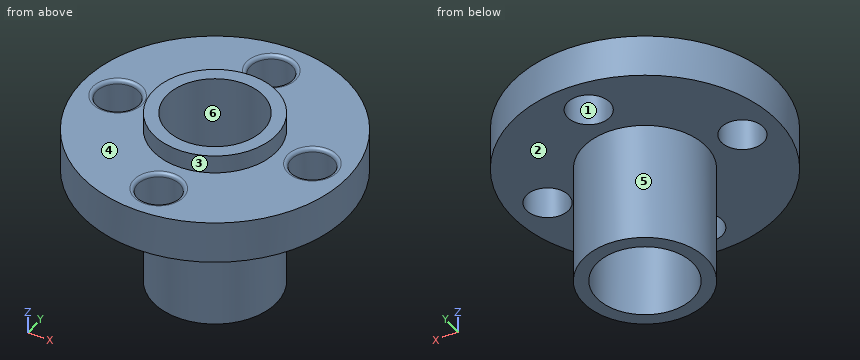
```python
from build123d import *

# Parameters (mm, degrees)
SKETCH1_R                = 11
SKETCH1_R_2              = 5.1
SKETCH1_R_3              = 1.75
BOSS_EXTRUDE1_DEPTH      = 3.5
BOSS_EXTRUDE2_DEPTH      = 1.5
BOSS_EXTRUDE2_DEPTH_BACK = 13.5
SKETCH2_R                = 5.1
SKETCH2_R_2              = 4
FILLET2_R                = 0.3


with BuildPart() as part:
    # Sketch1 → Boss-Extrude1 (new body)
    with BuildSketch(Plane.XY):
        Circle(SKETCH1_R)
        Circle(SKETCH1_R_2, mode=Mode.SUBTRACT)
        with Locations((0, 8)):
            Circle(SKETCH1_R_3, mode=Mode.SUBTRACT)
        with Locations((8, 0)):
            Circle(SKETCH1_R_3, mode=Mode.SUBTRACT)
        with Locations((0, -8)):
            Circle(SKETCH1_R_3, mode=Mode.SUBTRACT)
        with Locations((-8, 0)):
            Circle(SKETCH1_R_3, mode=Mode.SUBTRACT)
    extrude(amount=-BOSS_EXTRUDE1_DEPTH)

    # Sketch2 → Boss-Extrude2 (add, two sides: drawn at the far end of the back side and taken through both)
    with BuildSketch(Plane.XY.offset(-BOSS_EXTRUDE2_DEPTH_BACK)):
        Circle(SKETCH2_R)
        Circle(SKETCH2_R_2, mode=Mode.SUBTRACT)
    extrude(amount=BOSS_EXTRUDE2_DEPTH + BOSS_EXTRUDE2_DEPTH_BACK)

    # Fillet2
    fillet2_edges = [part.edges().sort_by_distance(p)[0] for p in [
        (6.25, 0, 0),
        (-1.75, -8, 0),
        (-9.75, 0, 0),
        (-1.75, 8, 0),
    ]]
    fillet(fillet2_edges, radius=FILLET2_R)


solid = part.part
```
The listing builds one solid part. Answer for the finished solid, in the listing's coordinates (mm). Face numbers are marked on the shaded views. A direction names the side the tool comes from. Round coordinates to 2 decimals unless told otherwise and drop trailing zeros. Order: outer loops, then holes, each group sorted by start corner. A loop starts at its lowest first (then second) coordinate and runs counter-clockwise, first axis right, second up. Notation, with made-up numbers: (-26.5, 43.5) - (12.5, 43.5) arc R33 ccw to (12.5, 74.5) - close; hole circle Ø11 at (33.25, 16). An arc over 180 degrees is marked (long way). Put each result on its own line as item: value. Start each with the question number.
(1) Straight lines are drawn through the part: probe 1 along Y at (x, z) = (0, -1.75); probe 2 along Z at (x, y) = (-4, 6.5); probe 3 along Y at (x, z) = (0, -8.5). For each, find the intervals that lie inside material, in ascending order. Write a range as from..to.
(2) Find section D-D (y = 8). Give the vertices of the cut face in (x, z), plus the area to 3 significant figures.
(3) Given P1, Ø2, axis at x = -1.5, y = 5, coming from the -Z side; P2, Ø6, axis at x = 8, z = -5.5, coming from the -Y side; P3, Ø8, axis at y = 3.5, z = -7, coming from the -X side; P4, Ø5.5, axis at x = 0, y = 8, coming from the -Z side, each flat-ended and moving along its own axis, determine where each tip first touches the part or whether it passes through.
(4) Determine the mould class of the marked faces 4, 5 and 6 for opening direction Y: released by +Y, released by -Y, zero draft, split by the parting line, or undercut.
(5) Find section C-C (z = -1). Give the vertices of the cut face in (x, y), plus the area to 3 significant figures.
(6) Find section A-A (y = 0). Give the vertices of the cut face in (x, z).
(7) For the marked faces 1, 2 and 3, determine the directions among +Z, -Z, +X, -X, +Y, -Y from which every point of the face is accessible in a straight line to the end or side of a thin tool.
Reply:
1. probe 1: -11..-9.75, -6.25..-4, 4..6.25, 9.75..11
1. probe 2: -3.5..0
1. probe 3: -5.1..-4, 4..5.1
2. outline: (-7.55, -3.5) - (-1.75, -3.5) - (-1.75, -0.3) arc R0.3 ccw to (-2.05, 0) - (-7.55, 0) - close; (1.75, -3.5) - (7.55, -3.5) - (7.55, 0) - (2.05, 0) arc R0.3 ccw to (1.75, -0.3) - close
2. area: 40.6 mm^2
3. P1: z = -13.5
3. P2: y = -9.37
3. P3: x = -10.89
3. P4: z = -3.5
4. face 4: zero draft
4. face 5: split by the parting line
4. face 6: undercut
5. outline: circle Ø22 at (0, 0); hole circle Ø3.5 at (-8, 0); hole circle Ø8 at (0, 0); hole circle Ø3.5 at (0, -8); hole circle Ø3.5 at (0, 8); hole circle Ø3.5 at (8, 0)
5. area: 291 mm^2
6. outline: (-11, -3.5) - (-9.75, -3.5) - (-9.75, -0.3) arc R0.3 ccw to (-10.05, 0) - (-11, 0) - close; (-6.25, -3.5) - (-5.1, -3.5) - (-5.1, -13.5) - (-4, -13.5) - (-4, 1.5) - (-5.1, 1.5) - (-5.1, 0) - (-5.95, 0) arc R0.3 ccw to (-6.25, -0.3) - close; (4, -13.5) - (5.1, -13.5) - (5.1, -3.5) - (6.25, -3.5) - (6.25, -0.3) arc R0.3 ccw to (5.95, 0) - (5.1, 0) - (5.1, 1.5) - (4, 1.5) - close; (9.75, -3.5) - (11, -3.5) - (11, 0) - (10.05, 0) arc R0.3 ccw to (9.75, -0.3) - close
7. face 1: +Z, -Z
7. face 2: -Z
7. face 3: +Z
